Verification items for this drawing (mm, ordinates from the low corner). A direction names the side the tool comes from. Round coordinates to 2 decimals unless told otherwise and drop trailing zeros. Order: outer loops, then holes, each group sorted by start corner. A loop starts at its lowest first (then second) coordinate and runs counter-clockwise, first axis right, second up. Notation, with made-up numbers: (10, 1.5) - (41, 1.5) arc R26 cw to (41, 17.5) - close; hole circle Ø3 at (-8.75, 71.25). An arc over 180 degrees is marked (long way). Use a Markdown table: item, result. Add a question column.
(1) Thickness scan on line 1 along Y through (x, z) = (234, 117); line 2 along Y through (x, z) = (190, 149); line 3 along X through (y, z) = (57.5, 138). Record the ranges inside material, lowest first. Write a range as [from, to].
(2) Section check C-C on z = 21. Record the boundary of the cut face in (x, y).
(3) Mould release check, pull along X, two halves, no side actions. Record for the marked faces 3, 4 and 5: released by +X, released by -X, zero draft, split by the parting line, or undercut.
(4) Gauge pin test, flat ends, axial feed: P1, Ø1, axis at x = 186.5, y = 50.5, coming from the -Z side; P2, Ø7.5, axis at y = 76.2, z = 76.2, coming from the +X side. Record the tip position at first contact, or that the pin passes through.
(5) Access from +Z, -Z, +X, -X, +Y, -Y to the whole of each face (thin tool, end or side, straight path). Record for the marked faces 1 and 2.
(6) Section check B-B on x = 114.3. Record the boundary of the cut face in (y, z), then the cut area to 3 significant figures.
(7) Section check A-A on y = 76.2. Record the boundary of the cut face in (x, z).
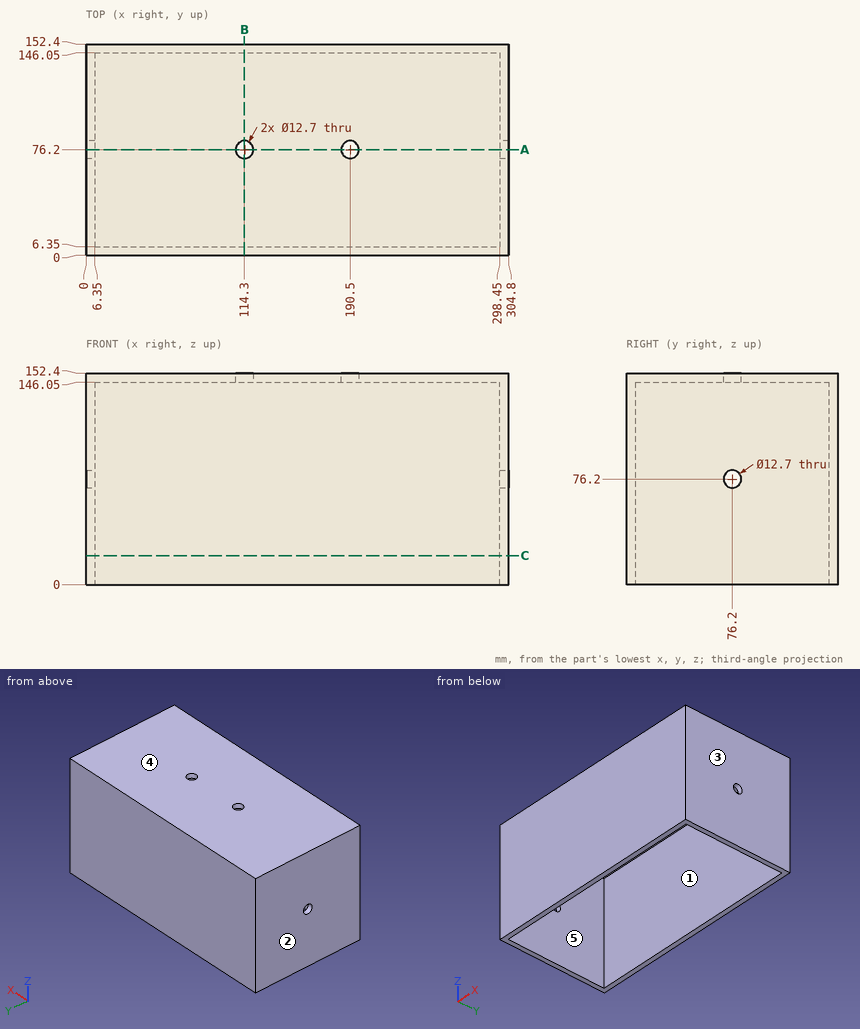
Check sheet entries:
| question | item | result |
|---|---|---|
| 1 | line 1 | y = [0, 6.35], [146.05, 152.4] |
| 1 | line 2 | y = [0, 69.87], [82.53, 152.4] |
| 1 | line 3 | x = [0, 6.35], [298.45, 304.8] |
| 2 | outline | (0, 0) - (304.8, 0) - (304.8, 152.4) - (0, 152.4) - close; hole (6.35, 6.35) - (298.45, 6.35) - (298.45, 146.05) - (6.35, 146.05) - close |
| 3 | face 3 | released by +X |
| 3 | face 4 | zero draft |
| 3 | face 5 | undercut |
| 4 | P1 | stops at z = 146.05 |
| 4 | P2 | passes through |
| 5 | face 1 | -Z |
| 5 | face 2 | +Z, -Z, -X, +Y, -Y |
| 6 | outline | (0, 0) - (6.35, 0) - (6.35, 146.05) - (69.85, 146.05) - (69.85, 152.4) - (0, 152.4) - close; (82.55, 146.05) - (146.05, 146.05) - (146.05, 0) - (152.4, 0) - (152.4, 152.4) - (82.55, 152.4) - close |
| 6 | area | 2,740 mm2 |
| 7 | outline | (0, 0) - (6.35, 0) - (6.35, 69.85) - (0, 69.85) - close; (0, 82.55) - (6.35, 82.55) - (6.35, 146.05) - (107.95, 146.05) - (107.95, 152.4) - (0, 152.4) - close; (120.65, 146.05) - (184.15, 146.05) - (184.15, 152.4) - (120.65, 152.4) - close; (196.85, 146.05) - (298.45, 146.05) - (298.45, 82.55) - (304.8, 82.55) - (304.8, 152.4) - (196.85, 152.4) - close; (298.45, 0) - (304.8, 0) - (304.8, 69.85) - (298.45, 69.85) - close |
